Input: part model. Units: mm. Frame: model coordinates. Face numbers are marked on the shaded views. A direction names the side the tool comes from. Coordinates: 2 decimals unless noted, no trailing zeros. Order: outer loops, then holes, each group sorted by start corner. A loop starts at its lowest first (then second) coordinate and runs counter-clockwise, first axis right, second up. Notation, with made-up numbers: (-6.75, -39.5) -> (36.25, -39.5) arc R7 cw to (36.25, -27.5) -> close; hole circle Ø5 at (-29, 45). An arc over 180 degrees is marked (long way). Answer as CSV lines item,"result".
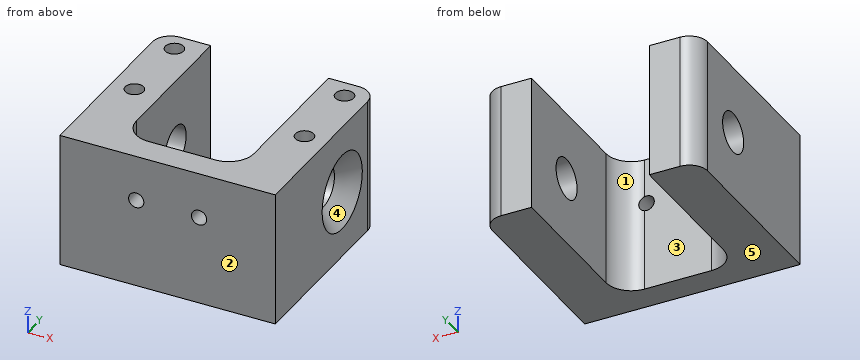
from build123d import *

# Parameters (mm, degrees)
SKETCH1_W                                           = 35.3
SKETCH1_H                                           = 22.1
BOSS_EXTRUDE1_DEPTH                                 = 32
SKETCH2_W                                           = 19.3
SKETCH2_H                                           = 27.52
CUT_EXTRUDE1_DEPTH                                  = 32
BOSS_EXTRUDE2_DEPTH                                 = 22.1
FILLET1_R                                           = 3
CSK_FOR_M6_COUNTERSUNK_FLAT_HEAD_SCREW1_D           = 6.6
CSK_FOR_M6_COUNTERSUNK_FLAT_HEAD_SCREW1_DEPTH       = 45
CSK_FOR_M6_COUNTERSUNK_FLAT_HEAD_SCREW1_CSINK_D     = 12.6
CSK_FOR_M6_COUNTERSUNK_FLAT_HEAD_SCREW1_CSINK_ANGLE = 90
CSK_FOR_M6_COUNTERSUNK_FLAT_HEAD_SCREW1_TIP         = 1.982840043
F_3_0MM_DOWEL_HOLE1_D                               = 3
F_3_0MM_DOWEL_HOLE1_DEPTH                           = 10
F_3_0MM_DOWEL_HOLE1_TIP                             = 0.901290929
F_2_5MM_DOWEL_HOLE1_D                               = 2.5
F_2_5MM_DOWEL_HOLE1_DEPTH                           = 10
F_2_5MM_DOWEL_HOLE1_TIP                             = 0.751075774


with BuildPart() as part:
    # Sketch1 → Boss-Extrude1 (new body)
    with BuildSketch(Plane(origin=(0, 0, 0), x_dir=(1, 0, 0), z_dir=(0, 1, 0))):
        with Locations((17.65, 11.05)):
            Rectangle(SKETCH1_W, SKETCH1_H)
    extrude(amount=BOSS_EXTRUDE1_DEPTH)

    # Sketch2 → Cut-Extrude1 (cut)
    with BuildSketch(Plane.XY):
        with Locations((17.65, 18.24)):
            Rectangle(SKETCH2_W, SKETCH2_H)
    extrude(amount=-CUT_EXTRUDE1_DEPTH, mode=Mode.SUBTRACT)

    # Sketch3 → Boss-Extrude2 (add)
    with BuildSketch(Plane.XY):
        with BuildLine():
            Line((8, 8.63), (8, 4.48))
            Line((8, 4.48), (12.15, 4.48))
            ThreePointArc((12.15, 4.48), (9.215506858, 5.695506858), (8, 8.63))
        make_face()
        with BuildLine():
            Line((27.3, 4.48), (27.3, 8.63))
            ThreePointArc((27.3, 8.63), (26.084493142, 5.695506858), (23.15, 4.48))
            Line((23.15, 4.48), (27.3, 4.48))
        make_face()
    extrude(amount=-BOSS_EXTRUDE2_DEPTH)

    # Fillet1
    fillet1_edges = [part.edges().sort_by_distance(p)[0] for p in [
        (35.3, 32, -11.05),
        (0, 32, -11.05),
    ]]
    fillet(fillet1_edges, radius=FILLET1_R)

    # CSK for M6 Countersunk Flat Head Screw1
    with Locations(Plane(origin=(35.3, 0, 0), x_dir=(0, 0, -1), z_dir=(1, 0, 0))):
        with Locations((11.1, 21)):
            CounterSinkHole(CSK_FOR_M6_COUNTERSUNK_FLAT_HEAD_SCREW1_D / 2, CSK_FOR_M6_COUNTERSUNK_FLAT_HEAD_SCREW1_CSINK_D / 2, depth=CSK_FOR_M6_COUNTERSUNK_FLAT_HEAD_SCREW1_DEPTH, counter_sink_angle=CSK_FOR_M6_COUNTERSUNK_FLAT_HEAD_SCREW1_CSINK_ANGLE)
            with Locations((0, 0, -(CSK_FOR_M6_COUNTERSUNK_FLAT_HEAD_SCREW1_DEPTH + CSK_FOR_M6_COUNTERSUNK_FLAT_HEAD_SCREW1_TIP / 2))):  # 118° drill point
                Cone(0, CSK_FOR_M6_COUNTERSUNK_FLAT_HEAD_SCREW1_D / 2, CSK_FOR_M6_COUNTERSUNK_FLAT_HEAD_SCREW1_TIP, mode=Mode.SUBTRACT)

    # Ø3.0mm Dowel Hole1
    with Locations(Plane.XY):
        with Locations((3.71, 28.82), (3.71, 16.26), (31.59, 28.82), (31.59, 16.26)):
            Hole(F_3_0MM_DOWEL_HOLE1_D / 2, depth=F_3_0MM_DOWEL_HOLE1_DEPTH)
            with Locations((0, 0, -(F_3_0MM_DOWEL_HOLE1_DEPTH + F_3_0MM_DOWEL_HOLE1_TIP / 2))):  # 118° drill point
                Cone(0, F_3_0MM_DOWEL_HOLE1_D / 2, F_3_0MM_DOWEL_HOLE1_TIP, mode=Mode.SUBTRACT)

    # Ø2.5mm Dowel Hole1
    with Locations(Plane(origin=(0, 0, 0), x_dir=(-1, 0, 0), z_dir=(0, -1, 0))):
        with Locations((-12.5, 7.5), (-22.8, 7.5)):
            Hole(F_2_5MM_DOWEL_HOLE1_D / 2, depth=F_2_5MM_DOWEL_HOLE1_DEPTH)
            with Locations((0, 0, -(F_2_5MM_DOWEL_HOLE1_DEPTH + F_2_5MM_DOWEL_HOLE1_TIP / 2))):  # 118° drill point
                Cone(0, F_2_5MM_DOWEL_HOLE1_D / 2, F_2_5MM_DOWEL_HOLE1_TIP, mode=Mode.SUBTRACT)


solid = part.part
1. Cut plane C-C (y = 6.5). Return the cut outline in (x, z), plus the area to 3 significant figures.
Findings:
outline,"(0, -22.1) -> (8.59, -22.1) -> (8.59, 0) -> (0, 0) -> close; (26.71, -22.1) -> (35.3, -22.1) -> (35.3, 0) -> (26.71, 0) -> close"
area,"380 mm2"
2. Ray query, line 1 along X through (y, z) = (28.82, -2.75); line 2 along Z through (x, y) = (12.5, 2.1); line 3 along X through (y, z) = (30, -6). Return the intervals inside material, ascending.
Findings:
line 1,"x = 0 to 2.21, 5.21 to 8, 27.3 to 30.09, 33.09 to 35.3"
line 2,"z = -22.1 to -8.75, -6.25 to 0"
line 3,"x = 0.17 to 2.78, 4.64 to 8, 27.3 to 30.66, 32.52 to 35.13"
3. Reachability of the marked faces 1 and 2 from +Z, -Z, +X, -X, +Y, -Y: full face, straight path, thin tool, end or side. Return the list, or none.
Findings:
face 1,"+Z, -Z, +Y"
face 2,"+Z, -Z, +X, -X, -Y"
4. Cut plane D-D (x = 18.5). Return the cut outline in (y, z).
Findings:
outline,"(0, -22.1) -> (4.48, -22.1) -> (4.48, 0) -> (0, 0) -> close"
5. Mould query, pull axis Y, two halves, no side actions, for the marked faces 3, 4 and 5. Classes: released by +Y, released by -Y, zero draft, split by the parting line, or undercut.
Findings:
face 3,"released by +Y"
face 4,"undercut"
face 5,"zero draft"
6. Cut plane B-B (z = -3.5). Return the cut outline in (x, y), plus the area to 3 significant figures.
Findings:
outline,"(0, 0) -> (35.3, 0) -> (35.3, 29) arc R3 ccw to (32.3, 32) -> (27.3, 32) -> (27.3, 8.63) arc R4.15 cw to (23.15, 4.48) -> (12.15, 4.48) arc R4.15 cw to (8, 8.63) -> (8, 32) -> (3, 32) arc R3 ccw to (0, 29) -> close; hole circle Ø3 at (3.71, 16.26); hole circle Ø3 at (3.71, 28.82); hole circle Ø3 at (31.59, 16.26); hole circle Ø3 at (31.59, 28.82)"
area,"574 mm2"
7. Cut plane A-A (y = 21). Return the cut outline in (x, z).
Findings:
outline,"(0, -22.1) -> (8, -22.1) -> (8, -14.4) -> (0, -14.4) -> close; (0, -7.8) -> (8, -7.8) -> (8, 0) -> (0, 0) -> close; (27.3, -22.1) -> (35.3, -22.1) -> (35.3, -17.4) -> (32.3, -14.4) -> (27.3, -14.4) -> close; (27.3, -7.8) -> (32.3, -7.8) -> (35.3, -4.8) -> (35.3, 0) -> (27.3, 0) -> close"
8. Contact query for flat-ended pins moving along their axis: pin 1 (1.5 mm diameter, centred on x = 12.5, z = -7.5, fed in from -Y); pin 2 (4 mm diameter, centred on x = 10.5, z = -13, fed in from +Y); pin 3 (4 mm diameter, centred on x = 22.8, z = -7.5, fed in from -Y); pin 4 (1.8 mm diameter, centred on x = 31.59, y = 16.26, fed in from +Z). Output: stop coordinate, or through.
Findings:
pin 1,"passes through"
pin 2,"stops at y = 6.66"
pin 3,"stops at y = 0"
pin 4,"stops at z = -10.36"
